Answer from the drawing. Dimensions are ordinates in mm from the lowest x, y and z of the part. Give positions to 0.01 mm unless a question says otherwise; leave off trailing zeros. Write each loop counter-clockwise with the first axis right and the second up, starting at its lowest first coordinate (ties: lowest second). Pieces come first, ordered by that corner, then holes. Notation, with made-up numbers: M 68.5,25.5 L 96.5,25.5 A32 cw 96.5,62.5 Z; hole C 69.5,36.25 d4. An arc over 180 degrees is marked long. Answer as a JSON object with one key per item and string values.
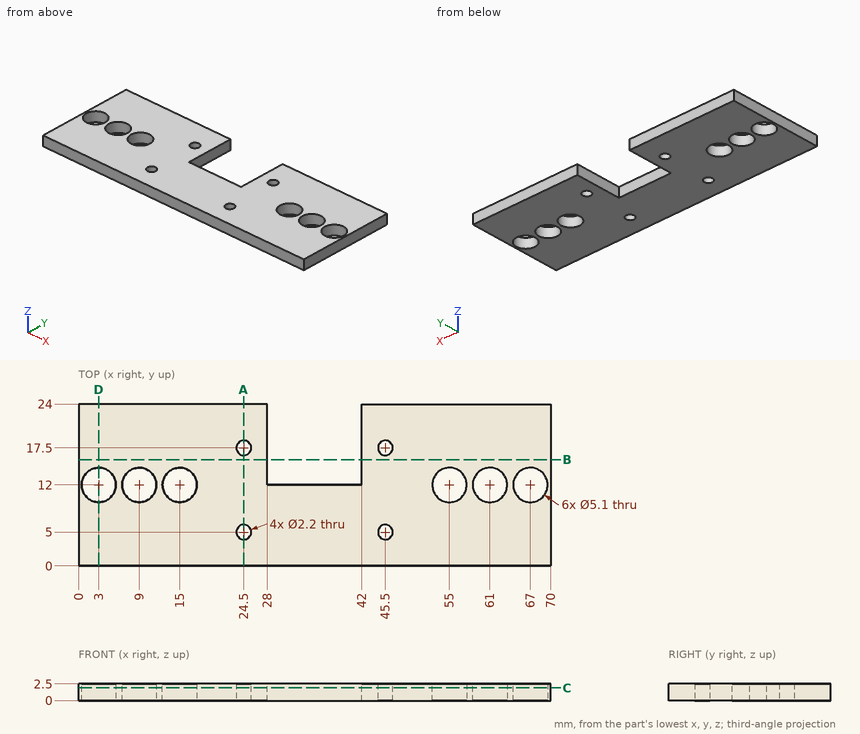
1. Consider line 1 along Y through (x, z) = (24.5, 0.8); line 2 along Y through (x, z) = (67, 1.3); line 3 along X through (y, z) = (4.5, 0.9). Determine where each line is inside the solid, lowest interval first.
Verdict:
{"line 1": "y = 0 to 3.9, 6.1 to 16.4, 18.6 to 24", "line 2": "y = 0 to 9.45, 14.55 to 24", "line 3": "x = 0 to 23.52, 25.48 to 44.52, 46.48 to 70"}
2. A cutting plane is placed at C-C, the plane z = 1.9. Count the separate pieces of the cut face and the enclosed holes in it, plus the area to 3 significant figures.
Verdict:
{"separate pieces": "1", "enclosed holes": "10", "area": "1,370 mm2"}
3. A cutting plane is placed at D-D, the plane x = 3. Give the vertices of the cut face in (y, z), plus the area to 4 significant figures.
Verdict:
{"outline": "M 0,0 L 9.45,0 L 9.45,2.5 L 0,2.5 Z; M 14.55,0 L 24,0 L 24,2.5 L 14.55,2.5 Z", "area": "47.25 mm2"}
4. A cutting plane is placed at A-A, the plane x = 24.5. Give the vertices of the cut face in (y, z), plus the area to 3 significant figures.
Verdict:
{"outline": "M 0,0 L 3.9,0 L 3.9,2.5 L 0,2.5 Z; M 6.1,0 L 16.4,0 L 16.4,2.5 L 6.1,2.5 Z; M 18.6,0 L 24,0 L 24,2.5 L 18.6,2.5 Z", "area": "49.0 mm2"}
5. A cutting plane is placed at B-B, the plane y = 15.75. Give the vertices of the cut face in (x, z), plus the area to 3 significant figures.
Verdict:
{"outline": "M 0,0 L 28,0 L 28,2.5 L 0,2.5 Z; M 42,0 L 70,0 L 70,2.5 L 42,2.5 Z", "area": "140 mm2"}
